Check sheet for the modelled part. Datum: model origin and axes. Units: mm. A direction names the side the tool comes from. Coordinates: 2 decimals unless noted, no trailing zeros. Write each loop counter-clockwise with the first axis right and the second up, starting at its lowest first coordinate (ties: lowest second). Pieces come first, ordered by that corner, then holes. Notation, with made-up numbers: (55, 8) - (101, 8) arc R23 ccw to (101, 34) - close; hole circle Ø7 at (-7.5, 11.25). An arc over 180 degrees is marked (long way). Write each question's results on one line, items separated by ' | '.
from build123d import *

# Parameters (mm, degrees)
SKETCH_1_W          = 30
SKETCH_1_H          = 120
EXTRUDE_1_DEPTH     = 10
SKETCH_2_W          = 30
SKETCH_2_H          = 114
CUT_EXTRUDE_1_DEPTH = 7
SKETCH_3_R          = 1.6
CUT_EXTRUDE_2_DEPTH = 121


with BuildPart() as part:
    # 草图1 → 凸台-拉伸1 (new body)
    with BuildSketch(Plane.XY):
        with Locations((4.914157805, 54.268009127)):
            Rectangle(SKETCH_1_W, SKETCH_1_H)
    extrude(amount=EXTRUDE_1_DEPTH)

    # 草图2 → 切除-拉伸1 (cut)
    with BuildSketch(Plane.XY.offset(10)):
        with Locations((4.914157805, 54.268009127)):
            Rectangle(SKETCH_2_W, SKETCH_2_H)
    extrude(amount=-CUT_EXTRUDE_1_DEPTH, mode=Mode.SUBTRACT)

    # 草图3 → 切除-拉伸2 (cut, through all)
    with BuildSketch(Plane(origin=(0, 114.268009127, 0), x_dir=(1, 0, 0), z_dir=(0, 1, 0))):
        with Locations((-5.085842195, -6)):
            Circle(SKETCH_3_R)
        with Locations((14.914157805, -6)):
            Circle(SKETCH_3_R)
    extrude(amount=-CUT_EXTRUDE_2_DEPTH, mode=Mode.SUBTRACT)


solid = part.part
1. Draft check along X on faces 1 (the cylindrical face through (16.392, 112.789, 6.613)), 2 (the flat face through (5, -5.732, 5)), 3 (the flat face through (19.914, 54, 2)), 4 (the cylindrical face through (16.392, -4.211, 6.613)). Enter one of: pulls with the +X half, pulls with the -X half, needs draft (parallel to the pull), parting line crosses it, or undercut.
Values follow:
face 1: undercut | face 2: needs draft | face 3: pulls with the +X half | face 4: undercut
2. Sectioned sample at A-A (z = 6). Record the cut outline in (x, y).
Values follow:
outline: (-10.09, -5.73) - (-6.69, -5.73) - (-6.69, -2.73) - (-10.09, -2.73) - close; (-10.09, 111.27) - (-6.69, 111.27) - (-6.69, 114.27) - (-10.09, 114.27) - close; (-3.49, -5.73) - (13.31, -5.73) - (13.31, -2.73) - (-3.49, -2.73) - close; (-3.49, 111.27) - (13.31, 111.27) - (13.31, 114.27) - (-3.49, 114.27) - close; (16.51, -5.73) - (19.91, -5.73) - (19.91, -2.73) - (16.51, -2.73) - close; (16.51, 111.27) - (19.91, 111.27) - (19.91, 114.27) - (16.51, 114.27) - close
3. Go/stop test with flat-tipped pins: pin 1 (3 mm diameter, centred on x = 14.91, z = 6, fed in from -Y); pin 2 (15 mm diameter, centred on x = 1, y = 42.5, fed in from +Z). Record where each tip stops, or that it passes through.
Values follow:
pin 1: passes through | pin 2: stops at z = 3
4. Access from +Z, -Z, +X, -X, +Y, -Y to the whole of each face (thin tool, end or side, straight path). Record for faces 5 (the flat face through (5, 111.268, 7)), 6 (the flat face through (5, 55, 0)).
Values follow:
face 5: +Z, +X, -X | face 6: -Z, +X, -X, +Y, -Y
5. Material ranges on L1, parallel to X at y = 113.4, z = 6; L2, parallel to Y at x = 12.5, z = 6; L3, parallel to Z at x = -3, y = 13, recorded low to high. Write a range as [from, to].
Values follow:
L1: x = [-10.09, -6.69], [-3.49, 13.31], [16.51, 19.91] | L2: y = [-5.73, -2.73], [111.27, 114.27] | L3: z = [0, 3]
6. Sectioned sample at C-C (y = 28). Record the cut outline in (x, z).
Values follow:
outline: (-10.09, 0) - (19.91, 0) - (19.91, 3) - (-10.09, 3) - close
7. Sectioned sample at B-B (x = -0.5). Record the cut outline in (y, z), then the cut area to 3 significant figures.
Values follow:
outline: (-5.73, 0) - (114.27, 0) - (114.27, 10) - (111.27, 10) - (111.27, 3) - (-2.73, 3) - (-2.73, 10) - (-5.73, 10) - close | area: 402 mm^2
